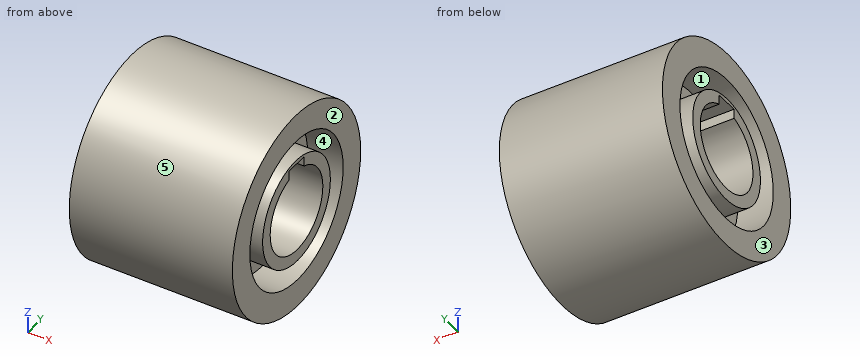
Solid Edge part; units mm, degrees
sketch "Sketch1" plane through (0, 0, 0) normal (1, 0, 0) x (0, 1, 0)
  circle A0 centre (0, 0) radius 17.5
  circle A1 centre (0, 0) radius 42.625
extrude "Protrusion1" add sketch "Sketch1" along normal mid plane 69
sketch "Sketch2" plane through (-34.5, 0, 0) normal (-1, 0, 0) x (0, -1, 0)
  circle A0 centre (0, 0) radius 22.5
  circle A1 centre (0, 0) radius 31
extrude "VaciadoExtruido_1" cut sketch "Sketch2" against normal blind 15
sketch "Sketch3" plane through (34.5, 0, 0) normal (1, 0, 0) x (0, 1, 0)
  circle A0 centre (0, 0) radius 22.5
  circle A1 centre (0, 0) radius 31
extrude "Cutout1" cut sketch "Sketch3" against normal blind 15
sketch "Sketch4" plane through (34.5, 0, 0) normal (1, 0, 0) x (0, 1, 0)
  line L0 (-5, 20.8) -> (-5, 16.7705)
  line L1 (0, 20.8) -> (-5, 20.8)
  line L2 (0, 20.8) -> (5, 20.8)
  line L3 (5, 20.8) -> (5, 16.7705)
  arc A0 (-5, 16.7705) -> (5, 16.7705) centre (0, 0) cw
extrude "VaciadoExtruido_36" cut sketch "Sketch4" along normal mid plane 264
properties material "Acero"
Design review of the part built by this model. Coordinates are the model's own, in mm. Face numbers are marked on the shaded views. A direction names the side the tool comes from. Give positions to 0.01 mm unless a question says otherwise; leave off trailing zeros. Order: outer loops, then holes, each group sorted by start corner. A loop starts at its lowest first (then second) coordinate and runs counter-clockwise, first axis right, second up. Notation, with made-up numbers: (40, -18) -> (63, -18) arc R28 cw to (63, 16) -> close; hole circle Ø9 at (-11.75, 47.25). An arc over 180 degrees is marked (long way). Write each question's results on one line, items separated by ' | '. Start each with the question number.
Q1. Add section A-A on x = 25. State how many separate pieces and enclosed holes the cut face has, and give its area (3 significant figures).
Q2. Wall thickness on L1, parallel to Z at x = -29.5, y = 0 (3 decimals); L2, parallel to Z at x = -3, y = 0 (3 decimals); L3, parallel to Z at x = -30.5, y = 3: over which ranges is each line inside the solid? List them lowest first. Write a range as from..to.
Q3. Mouldability with a two-part tool opening along Z and no side actions: class the marked faces 3, 4 and 5 as +Z half, -Z half, draft (parallel to the pull), parting line (faces both ways), or undercut.
Q4. Machinability: for the marked faces 1 and 2, which of the approach directions +Z, -Z, +X, -X, +Y, -Y give a long, thin tool a straight path to every point of the face, cutting with its end or side? Answer none if there is none.
Q5. For pin 1 (1 mm diameter, centred on x = 17.5, z = 24.5, fed in from -Y); pin 2 (3 mm diameter, centred on x = 27, y = -23.5, fed in from -Z); pin 3 (12 mm diameter, centred on x = 7.5, z = -10, fed in from -Y), all flat-tipped, find the tip position at first contact; note any pin that passes through.
Q6. Add section B-B on y = 0. Give the boundary of the cut face in (x, z) (3 decimals), and give its area (3 significant figures).
Q7. Add section C-C on z = 0. Give the boundary of the cut face in (x, y) (3 decimals), and give its area (3 significant figures).
Found:
1) separate pieces: 2 | enclosed holes: 2 | area: 3,280 mm2
2) L1: z = -42.625..-31, -22.5..-17.5, 20.8..22.5, 31..42.625 | L2: z = -42.625..-17.5, 20.8..42.625 | L3: z = -42.52..-30.85, -22.3..-17.24, 20.8..22.3, 30.85..42.52
3) face 3: draft | face 4: undercut | face 5: parting line
4) face 1: -X | face 2: +Z, -Z, +X, +Y, -Y
5) pin 1: stops at y = -35.23 | pin 2: stops at z = -36.51 | pin 3: stops at y = -42.44
6) outline: (-34.5, -42.625) -> (34.5, -42.625) -> (34.5, -31) -> (19.5, -31) -> (19.5, -22.5) -> (34.5, -22.5) -> (34.5, -17.5) -> (-34.5, -17.5) -> (-34.5, -22.5) -> (-19.5, -22.5) -> (-19.5, -31) -> (-34.5, -31) -> close; (-34.5, 20.8) -> (34.5, 20.8) -> (34.5, 22.5) -> (19.5, 22.5) -> (19.5, 31) -> (34.5, 31) -> (34.5, 42.625) -> (-34.5, 42.625) -> (-34.5, 31) -> (-19.5, 31) -> (-19.5, 22.5) -> (-34.5, 22.5) -> close | area: 2,730 mm2
7) outline: (-34.5, -42.625) -> (34.5, -42.625) -> (34.5, -31) -> (19.5, -31) -> (19.5, -22.5) -> (34.5, -22.5) -> (34.5, -17.5) -> (-34.5, -17.5) -> (-34.5, -22.5) -> (-19.5, -22.5) -> (-19.5, -31) -> (-34.5, -31) -> close; (-34.5, 17.5) -> (34.5, 17.5) -> (34.5, 22.5) -> (19.5, 22.5) -> (19.5, 31) -> (34.5, 31) -> (34.5, 42.625) -> (-34.5, 42.625) -> (-34.5, 31) -> (-19.5, 31) -> (-19.5, 22.5) -> (-34.5, 22.5) -> close | area: 2,960 mm2
